Verification items for the finished model (mm, model axes). Face numbers are marked on the shaded views. A direction names the side the tool comes from. Round coordinates to 2 decimals unless told otherwise and drop trailing zeros. Write each loop counter-clockwise with the first axis right and the second up, starting at its lowest first coordinate (ties: lowest second). Pieces come first, ordered by that corner, then holes. Notation, with made-up numbers: M -34.5,-11.75 L 24.5,-11.75 A27 ccw 24.5,24.25 Z; hole C -24,10.25 d5. An arc over 180 degrees is marked long. One line per question, with ' | ' between items.
from build123d import *

# Parameters (mm, degrees)
F1_DEPTH = 4.2
F3_DEPTH = 1
F5_DEPTH = 5.201
F6_SIZE  = 0.25


with BuildPart() as f1:
    # F0 (on Top) → F1 (new body)
    with BuildSketch(Plane.XY):
        with BuildLine():
            Line((19, 3), (-19, 3))
            ThreePointArc((-19, 3), (-22, 0), (-19, -3))
            Line((-19, -3), (19, -3))
            ThreePointArc((19, -3), (22, 0), (19, 3))
        make_face()
    extrude(amount=-F1_DEPTH)

    # F2 (on face) → F3 (join)
    with BuildSketch(Plane.XY):
        with BuildLine():
            ThreePointArc((-19, 5), (-24, 0), (-19, -5))
            Line((-19, -5), (19, -5))
            ThreePointArc((19, -5), (24, 0), (19, 5))
            Line((19, 5), (-19, 5))
        make_face()
    extrude(amount=F3_DEPTH)

    # F4 (on face) → F5 (cut, through all)
    with BuildSketch(Plane.XY.offset(1)):
        with BuildLine():
            Line((-19, -2.1), (19, -2.1))
            ThreePointArc((19, -2.1), (21.1, 0), (19, 2.1))
            Line((19, 2.1), (-19, 2.1))
            ThreePointArc((-19, 2.1), (-21.1, 0), (-19, -2.1))
        make_face()
    extrude(amount=-F5_DEPTH, mode=Mode.SUBTRACT)

    # F6
    f6_edges = [f1.edges().sort_by_distance(p)[0] for p in [
        (-24, 0, 1),
        (0, 5, 1),
        (0, -5, 1),
        (24, 0, 1),
        (0, -2.1, 1),
        (21.1, 0, 1),
        (0, 2.1, 1),
        (-21.1, 0, 1),
    ]]
    chamfer(f6_edges, length=F6_SIZE)


solid = f1.part
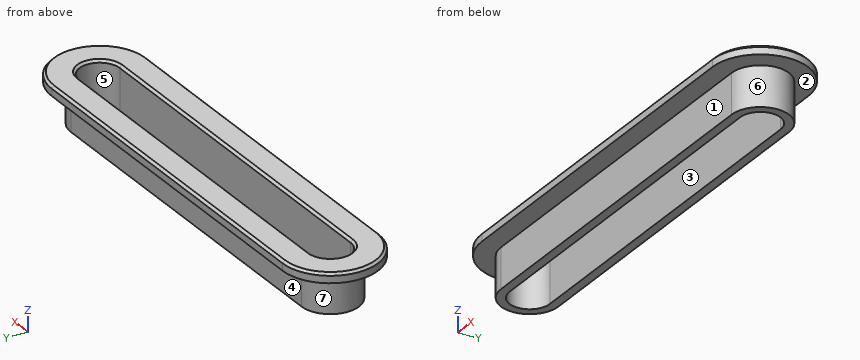
1. Go/stop test with flat-tipped pins: P1, Ø3, axis at x = 8.5, y = -0.5, coming from the -Z side; P2, Ø2, axis at x = 2, y = -3.5, coming from the -Z side; P3, Ø1.5, axis at x = -9, z = -1.5, coming from the +Y side; P4, Ø2.5, axis at x = -3, z = -3, coming from the -Y side. Record where each tip stops, or that it passes through.
Results:
P1: passes through | P2: stops at z = -4.2 | P3: stops at y = 3 | P4: stops at y = -3
2. Section check B-B, the plane z = -2.1. Record the cut outline in (x, y), then the cut area to 3 significant figures.
Results:
outline: M -19,-3 L 19,-3 A3 ccw 19,3 L -19,3 A3 ccw Z; hole M -19,-2.1 L 19,-2.1 A2.1 ccw 19,2.1 L -19,2.1 A2.1 ccw Z | area: 82.8 mm2
3. Section check A-A, the plane y = 0. Record the cut outline in (x, z).
Results:
outline: M -24,0 L -22,0 L -22,-4.2 L -21.1,-4.2 L -21.1,0.75 L -21.35,1 L -23.75,1 L -24,0.75 Z; M 21.1,-4.2 L 22,-4.2 L 22,0 L 24,0 L 24,0.75 L 23.75,1 L 21.35,1 L 21.1,0.75 Z
4. Mould release check, pull along Y, two halves, no side actions. Record for the marked faces 1, 2 and 3: pulls with the +Y half, pulls with the -Y half, needs draft (parallel to the pull), parting line crosses it, or undercut.
Results:
face 1: pulls with the -Y half | face 2: needs draft | face 3: undercut
5. Thickness scan on line 1 (Y direction, x = -18.5, z = -1); line 2 (X direction, y = 0.75, z = 0.6); line 3 (Z direction, x = 14, y = -3.5). Record the ranges inside material, lowest first.
Results:
line 1: y = -3 to -2.1, 2.1 to 3 | line 2: x = -23.94 to -20.96, 20.96 to 23.94 | line 3: z = 0 to 1
6. Tool access check on the marked faces 4, 5, 6 and 7. Record the directions out of +Z, -Z, +X, -X, +Y, -Y that give a thin tool (end or side, any length) a straight path to the whole face; none if there is none.
Results:
face 4: -Z, +X, -X, +Y | face 5: +Z, -Z | face 6: -Z, +X | face 7: -Z, -X
7. Section check C-C, the plane x = 15.5. Record the cut outline in (y, z).
Results:
outline: M -5,0 L -3,0 L -3,-4.2 L -2.1,-4.2 L -2.1,0.75 L -2.35,1 L -4.75,1 L -5,0.75 Z; M 2.1,-4.2 L 3,-4.2 L 3,0 L 5,0 L 5,0.75 L 4.75,1 L 2.35,1 L 2.1,0.75 Z
